Input: dimensioned drawing with shaded views. Units: mm. Origin: part minimum x, y, z. A direction names the side the tool comes from. Give positions to 0.01 mm unless a question says otherwise; leave off trailing zeros. Order: outer loops, then holes, each group sorted by start corner. A loop starts at its lowest first (then second) coordinate and runs counter-clockwise, first axis right, second up. Notation, with made-up numbers: (-15, -17.75) -> (23, -17.75) arc R27 cw to (23, 5.25) -> close; hole circle Ø1 at (-36, 56). An arc over 180 degrees is marked (long way). Use CSV: the item, a comma, the result in double quotes.
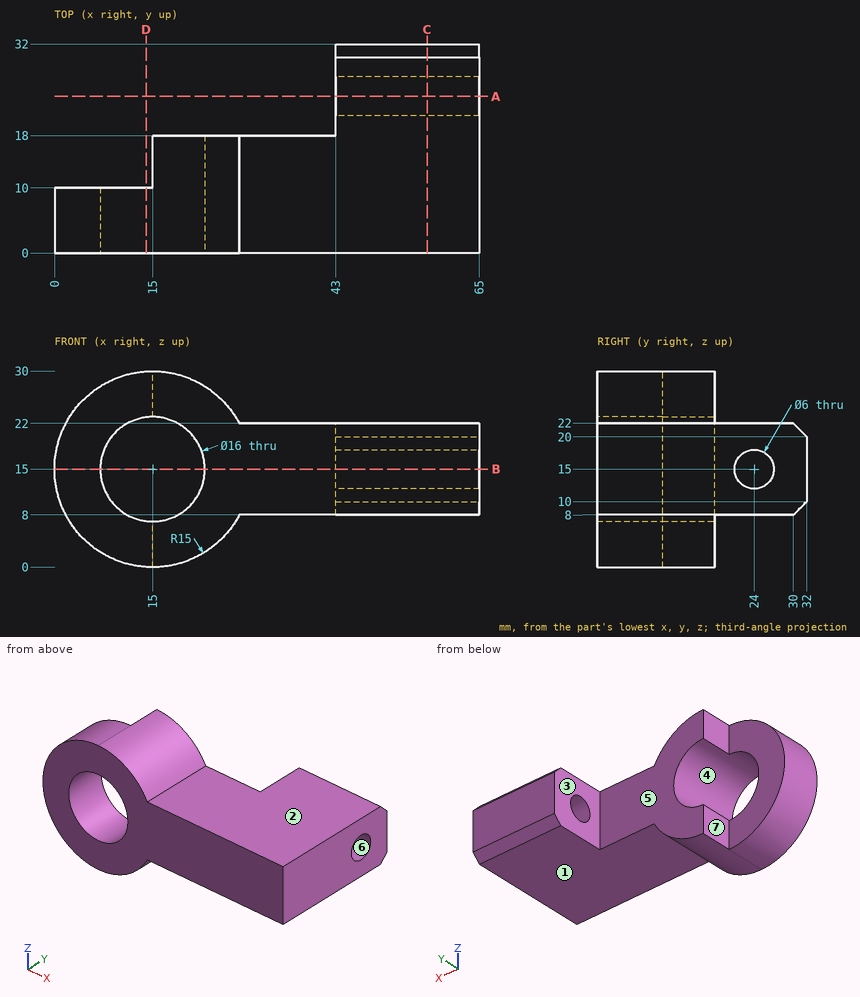
1. Section query D-D on x = 14. Return loops of the section in (y, z).
Answer below:
outline,"(0, 0.03) -> (10, 0.03) -> (10, 7.06) -> (0, 7.06) -> close; (0, 22.94) -> (10, 22.94) -> (10, 29.97) -> (0, 29.97) -> close"
2. Pin query (flat end, axial travel): P1, Ø2, axis at y = 13.5, z = 2.5, coming from the -X side; P2, Ø12, axis at y = 22.5, z = 17, coming from the -X side; P3, Ø9, axis at x = 41, y = 20, coming from the +Z side. Return the tip coordinate at first contact, or that it passes through.
Answer below:
P1,"stops at x = 15"
P2,"stops at x = 20.33"
P3,"stops at z = 22"
3. Ray query, line 1 along Z through (x, y) = (15, 9.25); line 2 along Y through (x, z) = (27, 21.5); line 3 along Y through (x, z) = (56, 15). Return the intervals inside material, ascending.
Answer below:
line 1,"z = 0 to 7, 23 to 30"
line 2,"y = 0 to 18"
line 3,"y = 0 to 21, 27 to 32"
4. Mould query, pull axis Y, two halves, no side actions, for the marked faces 5, 6 and 7. Classes: released by +Y, released by -Y, zero draft, split by the parting line, or undercut.
Answer below:
face 5,"released by +Y"
face 6,"undercut"
face 7,"zero draft"
5. Section query B-B on z = 15. Return loops of the section in (x, y).
Answer below:
outline,"(0, 0) -> (7, 0) -> (7, 10) -> (0, 10) -> close; (23, 0) -> (65, 0) -> (65, 21) -> (43, 21) -> (43, 18) -> (23, 18) -> close; (43, 27) -> (65, 27) -> (65, 32) -> (43, 32) -> close"
6. Section query C-C on x = 57. Return loops of the section in (y, z).
Answer below:
outline,"(0, 8) -> (30, 8) -> (32, 10) -> (32, 20) -> (30, 22) -> (0, 22) -> close; hole circle Ø6 at (24, 15)"
7. Section query A-A on y = 24. Return loops of the section in (x, z).
Answer below:
outline,"(43, 8) -> (65, 8) -> (65, 12) -> (43, 12) -> close; (43, 18) -> (65, 18) -> (65, 22) -> (43, 22) -> close"
8. Access query for the marked faces 1, 2, 3 and 4. Directions: +Z, -Z, +X, -X, +Y, -Y. A direction counts if a zero-diameter tool reaches every point of the face in a straight line with its end or side. Return the directions, or none.
Answer below:
face 1,"-Z, +X, +Y, -Y"
face 2,"+Z, +X, +Y, -Y"
face 3,"+Z, -Z, -X, +Y"
face 4,"+Y, -Y"
